Source: CAD feature listing. Evaluate the final solid. Frame: model axes, mm. Give positions to 0.01 mm unless a question says otherwise; leave off trailing zeros. Write each loop counter-clockwise with the first axis right and the second up, starting at its lowest first coordinate (ties: lowest second). Pieces come first, ordered by that corner, then holes. Notation, with made-up numbers: (51, 15.5) -> (99, 15.5) arc R18 cw to (99, 40.5) -> close; hole circle Ø10 at (6.25, 25). An arc over 180 degrees is marked (long way). Use a Markdown table: item, result. Add a question column.
```python
from build123d import *

# Parameters (mm, degrees)
SKETCH1_W           = 38.1
SKETCH1_H           = 19.05
BOSS_EXTRUDE1_DEPTH = 12.7


with BuildPart() as part:
    # Sketch1 → Boss-Extrude1 (new body)
    with BuildSketch(Plane.XY):
        Rectangle(SKETCH1_W, SKETCH1_H)
    extrude(amount=BOSS_EXTRUDE1_DEPTH)

    # Sketch2 → Revolve1 (revolve)
    with BuildSketch(Plane(origin=(0, 0, 0), x_dir=(0, 0, -1), z_dir=(1, 0, 0))):
        Polygon((0, 0), (-800, 953.402874075), (-800, 0), align=None)
    revolve(axis=Axis((0, 0, 800), (0, 0, -1)))


solid = part.part
```
(1) First-contact query: pin 1 Ø4 at (y, z) = (2.5, 9) entering from +X; pin 2 Ø4 at (x, y) = (-79, 755) entering from -Z; pin 3 Ø4 at (x, z) = (9.5, 7) entering from +Y (3 decimals). Flat tips, straight axial feed; report the tip coordinate or a pass-through.
(2) Cut plane A-A on z = 83. Return the cut outline in (x, y), then the cut area to 3 significant figures.
(3) Material intervals for L1, parallel to X at y = 462, z = 721.5; L2, parallel to X at y = 161.5, z = 613; L3, parallel to Y at x = 242, z = 242.5, sorted ascending.
(4) Cut plane B-B on z = 474. Return the cut outline in (x, y), then the cut area to 3 significant figures.
Output:
| question | item | result |
|---|---|---|
| 1 | pin 1 | x = 19.05 |
| 1 | pin 2 | z = 635.3 |
| 1 | pin 3 | y = 9.525 |
| 2 | outline | circle Ø197.83 at (0, 0) |
| 2 | area | 30,700 mm^2 |
| 3 | L1 | -725.19 to 725.19 |
| 3 | L2 | -712.47 to 712.47 |
| 3 | L3 | -157.98 to 157.98 |
| 4 | outline | circle Ø1129.78 at (0, 0) |
| 4 | area | 1,000,000 mm^2 |
